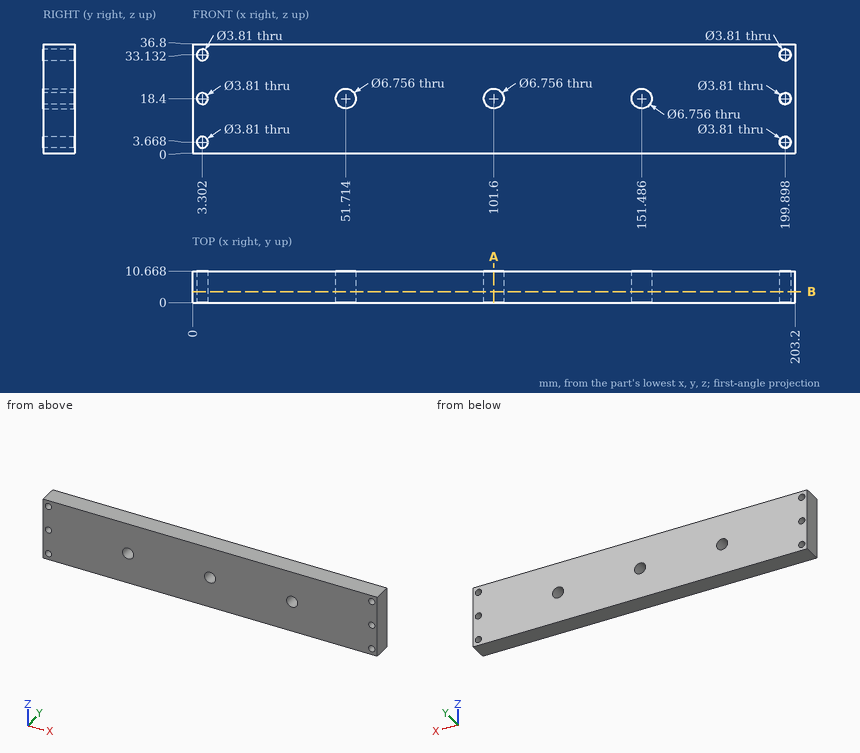
Input: dimensioned drawing with shaded views. Units: mm. Origin: part minimum x, y, z. Coordinates: 2 decimals unless noted, no trailing zeros. Write each loop counter-clockwise with the first axis right and the second up, starting at its lowest first coordinate (ties: lowest second). Pieces come first, ordered by that corner, then holes. Notation, with made-up numbers: (6.25, 11.25) -> (17.25, 11.25) arc R21 cw to (17.25, 40.25) -> close; hole circle Ø11 at (83.25, -4.5). An arc over 180 degrees is marked (long way). Return JSON: item names as keys, results as strings. Group by question number.
1) Section query A-A, the plane x = 101.6. Return loops of the section in (y, z).
2) Section query B-B, the plane y = 3.75. State how many separate pieces and enclosed holes the cut face has, plus the area to 3 significant figures.
3) Contact query for a flat-ended pin moving along its axis: P1, Ø5, axis at x = 3.3, z = 33.13, coming from the +Y side. Output: stop coordinate, or through.
4) Ray query, line 1 along X through (y, z) = (5.25, 33); line 2 along X through (y, z) = (0.75, 18) (1 decimal); line 3 along X through (y, z) = (7.5, 34) (1 decimal). Return the intervals inside material, ascending.
From the geometry:
{
 "1": {"outline": "(0, 0) -> (10.67, 0) -> (10.67, 15.02) -> (0, 15.02) -> close; (0, 21.78) -> (10.67, 21.78) -> (10.67, 36.8) -> (0, 36.8) -> close"},
 "2": {"separate pieces": "1", "enclosed holes": "9", "area": "7,300 mm²"},
 "3": {"P1": "y = 10.67"},
 "4": {"line 1": "0 to 1.4, 5.2 to 198, 201.8 to 203.2", "line 2": "0 to 1.4, 5.2 to 48.4, 55.1 to 98.2, 105 to 148.1, 154.8 to 198, 201.8 to 203.2", "line 3": "0 to 1.6, 5 to 198.2, 201.6 to 203.2"}
}
